Verification items for the finished model (mm, model axes). Coordinates: 2 decimals unless noted, no trailing zeros. Loops run counter-clockwise (first coordinate to the right, second up) from the corner with the lowest first, then second, coordinate; pieces in that order, holes last. Notation, with made-up numbers: (70.25, 66) -> (126.25, 66) arc R22 cw to (126.25, 91) -> close; hole circle Ø4 at (33.25, 43.5). An arc over 180 degrees is marked (long way). Use CSV: the item, a comma, the result in double quotes. Start each with the question number.
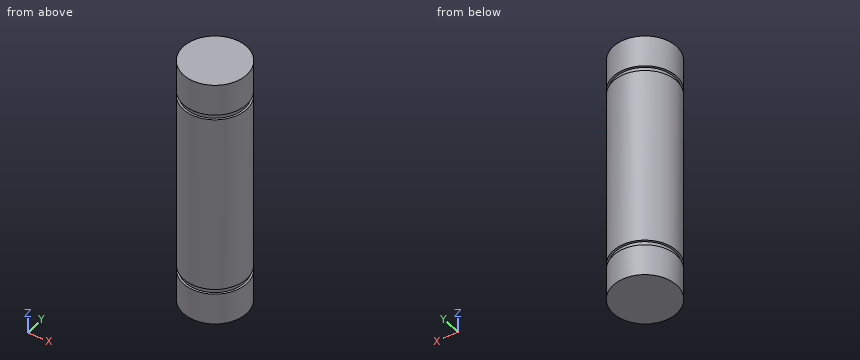
Autodesk Inventor part; units mm, degrees
ref_plane "YZ Plane" through (0, 0, 0) normal (1, 0, 0) x (0, 1, 0)
ref_plane "XZ Plane" through (0, 0, 0) normal (0, 1, 0) x (-1, 0, 0)
sketch "Sketch1" plane through (0, 0, 0) normal (0, 0, 1) x (1, 0, 0)
  circle A0 centre (0, 0) radius 6.35
  dimension "d0" = 12.7
extrude "Extrusion1" add sketch "Sketch1" along normal mid plane 50.8
ref_plane "Work Plane1" through (0, 0, 19.05) normal (0, 0, 1) x (1, 0, 0)
sketch "Sketch2" plane through (0, 0, 19.05) normal (0, 0, 1) x (1, 0, 0)
  circle A0 centre (0, 0) radius 6.35
  circle A1 centre (0, 0) radius 6.35
  circle A2 centre (0, 0) radius 5.9436
  dimension "d4" = 12.7
  dimension "d5" = 11.8872
extrude "Extrusion2" cut sketch "Sketch2" against normal blind 0.9906
mirror "Mirror1" about plane through (0, 0, 0) normal (0, 0, 1) of "Extrusion2"
ref_plane "Work Plane2" through (0, 0, -19.05) normal (0, 0, 1) x (1, 0, 0)
properties part number "Linear Actuator Top Pin .5in. Dia." material "Aluminum 6061"
1. Cross-section at B-B, the plane z = -14. Record the boundary of the cut face in (x, y).
2. Scan lines: line 1 (Z direction, x = 4.5, y = 4); line 2 (Y direction, x = 0.25, z = 16); line 3 (Y direction, x = 2.25, z = 21). Record each from-to range of solid material in increasing order.
3. Cross-section at A-A, the plane y = -3.5. Record the boundary of the cut face in (x, z).
4. Depth check by flat-ended pin: pin 1 (1.5 mm diameter, centred on y = 2.5, z = 4.5, fed in from +X); pin 2 (5 mm diameter, centred on x = 3, z = -6, fed in from +Y). Enter the tip coordinate at first touch or a pass-through.
5. Cross-section at C-C, the plane x = 4.75. Record the boundary of the cut face in (y, z), plus the area to 3 significant figures.
Solution:
1,outline,"circle Ø12.7 at (0, 0)"
2,line 1,"z = -25.4 to -19.05, -18.06 to 18.06, 19.05 to 25.4"
2,line 2,"y = -6.35 to 6.35"
2,line 3,"y = -5.94 to 5.94"
3,outline,"(-5.3, -25.4) -> (5.3, -25.4) -> (5.3, -19.05) -> (4.8, -19.05) -> (4.8, -18.06) -> (5.3, -18.06) -> (5.3, 18.06) -> (4.8, 18.06) -> (4.8, 19.05) -> (5.3, 19.05) -> (5.3, 25.4) -> (-5.3, 25.4) -> (-5.3, 19.05) -> (-4.8, 19.05) -> (-4.8, 18.06) -> (-5.3, 18.06) -> (-5.3, -18.06) -> (-4.8, -18.06) -> (-4.8, -19.05) -> (-5.3, -19.05) -> close"
4,pin 1,"stops at x = 6.1"
4,pin 2,"stops at y = 6.33"
5,outline,"(-4.21, -25.4) -> (4.21, -25.4) -> (4.21, -19.05) -> (3.57, -19.05) -> (3.57, -18.06) -> (4.21, -18.06) -> (4.21, 18.06) -> (3.57, 18.06) -> (3.57, 19.05) -> (4.21, 19.05) -> (4.21, 25.4) -> (-4.21, 25.4) -> (-4.21, 19.05) -> (-3.57, 19.05) -> (-3.57, 18.06) -> (-4.21, 18.06) -> (-4.21, -18.06) -> (-3.57, -18.06) -> (-3.57, -19.05) -> (-4.21, -19.05) -> close"
5,area,"426 mm2"
